Build history of the part. All positions in model axes, mm. Face numbers are marked on the shaded views. A direction names the side the tool comes from. Round coordinates to 2 decimals unless told otherwise and drop trailing zeros. Write each loop counter-clockwise with the first axis right and the second up, starting at its lowest first coordinate (ties: lowest second). Pieces come first, ordered by that corner, then holes. Notation, with made-up numbers: (8, -34) -> (31, -34) arc R25 ccw to (31, -16) -> close; hole circle Ø9 at (-6, 73). An arc over 180 degrees is marked (long way). Answer in a Markdown table with one row per item.
```python
from build123d import *

# Parameters (mm, degrees)
SKETCH1_W           = 52
SKETCH1_H           = 190
BOSS_EXTRUDE1_DEPTH = 15
SKETCH2_W           = 35
SKETCH2_H           = 54
CUT_EXTRUDE1_DEPTH  = 7.5
SKETCH4_W           = 36
SKETCH4_H           = 47
CUT_EXTRUDE7_DEPTH  = 5
SKETCH9_W           = 25
SKETCH9_H           = 25
CUT_EXTRUDE8_DEPTH  = 198.557586541
SKETCH5_W           = 7.5
SKETCH5_H           = 18
SKETCH5_H_2         = 15
CUT_EXTRUDE5_DEPTH  = 20


with BuildPart() as part:
    # Sketch1 → Boss-Extrude1 (new body)
    with BuildSketch(Plane.XY):
        with Locations((26, 95)):
            Rectangle(SKETCH1_W, SKETCH1_H)
    boss_extrude1 = extrude(amount=BOSS_EXTRUDE1_DEPTH)

    # Sketch2 → Cut-Extrude1 (cut)
    with BuildSketch(Plane.XY.offset(15)):
        with Locations((34.5, 97.5)):
            Rectangle(SKETCH2_W, SKETCH2_H)
    cut_extrude1 = extrude(amount=-CUT_EXTRUDE1_DEPTH, mode=Mode.SUBTRACT)

    # Sketch4 → Cut-Extrude7 (cut)
    with BuildSketch(Plane(origin=(0, 0, 0), x_dir=(-1, 0, 0), z_dir=(0, 0, -1))):
        with Locations((-52, 156.5)):
            Rectangle(SKETCH4_W, SKETCH4_H)
    cut_extrude7 = extrude(amount=-CUT_EXTRUDE7_DEPTH, mode=Mode.SUBTRACT)

    # Sketch9 → Cut-Extrude8 (cut, through all)
    with BuildSketch(Plane.XY.offset(15)):
        with Locations((12.5, 44.5)):
            Rectangle(SKETCH9_W, SKETCH9_H)
    cut_extrude8 = extrude(amount=-CUT_EXTRUDE8_DEPTH, mode=Mode.SUBTRACT)

    # Sketch5 → Cut-Extrude5 (cut)
    with BuildSketch(Plane(origin=(17, 0, 0), x_dir=(0, 0, -1), z_dir=(1, 0, 0))):
        with Locations((-11.25, 110.5)):
            Rectangle(SKETCH5_W, SKETCH5_H)
        with Locations((-11.25, 80)):
            Rectangle(SKETCH5_W, SKETCH5_H_2)
    extrude(amount=-CUT_EXTRUDE5_DEPTH, mode=Mode.SUBTRACT)

    # Mirror4: Boss-Extrude1, Cut-Extrude1, Cut-Extrude7, Cut-Extrude8 across plane
    add(boss_extrude1.mirror(Plane(origin=(52, 0, 0), x_dir=(0, 0, 1), z_dir=(1, 0, 0))))
    add(cut_extrude1.mirror(Plane(origin=(52, 0, 0), x_dir=(0, 0, 1), z_dir=(1, 0, 0))), mode=Mode.SUBTRACT)
    add(cut_extrude7.mirror(Plane(origin=(52, 0, 0), x_dir=(0, 0, 1), z_dir=(1, 0, 0))), mode=Mode.SUBTRACT)
    add(cut_extrude8.mirror(Plane(origin=(52, 0, 0), x_dir=(0, 0, 1), z_dir=(1, 0, 0))), mode=Mode.SUBTRACT)


solid = part.part
```
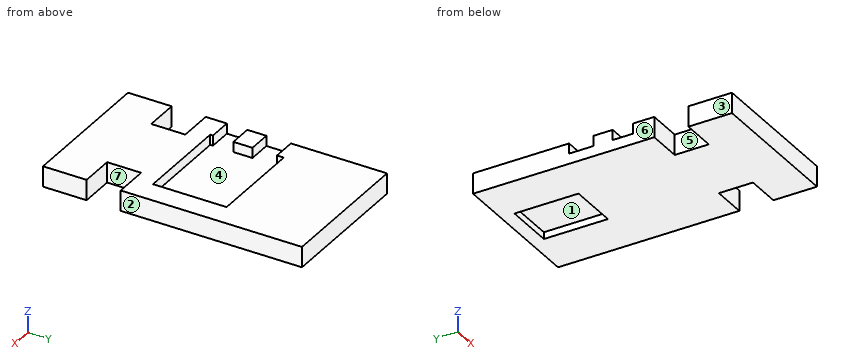
Q1. Two-plate mould, pull along X, no slides. Class the marked faces 1, 2, 3 and 4: released by +X, released by -X, zero draft, split by the parting line, or undercut.
A:
| item | result |
|---|---|
| face 1 | undercut |
| face 2 | released by +X |
| face 3 | released by -X |
| face 4 | undercut |
Q2. Which spindle directions (+Z, -Z, +X, -X, +Y, -Y) get a long thin tool onto all of the face, cutting with end or side? Do the marked faces 5, 6 and 7. Say none if no direction does.
A:
| item | result |
|---|---|
| face 5 | +Z, -Z, -X |
| face 6 | +Z, -Z, -X, +Y, -Y |
| face 7 | +Z, -Z, +X |
Q3. Saw through at C-C on y = 176. Write the cut outline in (x, z).
A:
| item | result |
|---|---|
| outline | (0, 0) -> (34, 0) -> (34, 5) -> (70, 5) -> (70, 0) -> (104, 0) -> (104, 15) -> (0, 15) -> close |
Q4. Saw through at D-D on x = 11. Write the cut outline in (y, z).
A:
| item | result |
|---|---|
| outline | (0, 0) -> (32, 0) -> (32, 15) -> (0, 15) -> close; (57, 0) -> (190, 0) -> (190, 15) -> (119.5, 15) -> (119.5, 7.5) -> (101.5, 7.5) -> (101.5, 15) -> (87.5, 15) -> (87.5, 7.5) -> (72.5, 7.5) -> (72.5, 15) -> (57, 15) -> close |
Q5. Saw through at B-B on z = 2.5. Write the cut outline in (x, y).
A:
| item | result |
|---|---|
| outline | (0, 0) -> (104, 0) -> (104, 32) -> (79, 32) -> (79, 57) -> (104, 57) -> (104, 190) -> (0, 190) -> (0, 57) -> (25, 57) -> (25, 32) -> (0, 32) -> close; hole (34, 133) -> (70, 133) -> (70, 180) -> (34, 180) -> close |
Q6. Wall check: line 1 (Y direction, x = 79.5, z = 9); line 2 (Y direction, x = 67, z = 10.5); line 3 (Y direction, x = 12, z = 7). Give the ranges that are in metal, low to high. Write a range as [from, to].
A:
| item | result |
|---|---|
| line 1 | [0, 32], [57, 70.5], [124.5, 190] |
| line 2 | [0, 70.5], [124.5, 190] |
| line 3 | [0, 32], [57, 190] |
Q7. Drop flat-ended pins along their axis: P1, Ø2, axis at y = 112.5, z = 13, coming from the -X side; P2, Ø4, axis at x = 36.5, y = 88.5, coming from the +Z side; P3, Ø7.5, axis at y = 44.5, z = 5.5, coming from the -X side. Give the stop position or say it passes through.
A:
| item | result |
|---|---|
| P1 | x = 87 |
| P2 | z = 7.5 |
| P3 | x = 25 |
Q8. Saw through at A-A on x = 90. Write the cut outline in (y, z), plus the area to 4 significant figures.
A:
| item | result |
|---|---|
| outline | (0, 0) -> (32, 0) -> (32, 15) -> (0, 15) -> close; (57, 0) -> (190, 0) -> (190, 15) -> (57, 15) -> close |
| area | 2,475 mm² |
